```python
from build123d import *

# Parameters (mm, degrees)
FILLET1_R    = 2.1
SCALE1_SCALE = 1.2
SCALE2_SCALE = 0.1


with BuildPart() as part:
    # Sketch1 → Revolve1 (revolve)
    with BuildSketch(Plane.XY):
        with BuildLine():
            Line((-15.5, 65), (15.5, 65))
            Line((15.5, 65), (15.5, 53))
            Line((15.5, 53), (8.94427191, 53))
            ThreePointArc((8.94427191, 53), (0, 57), (-8.94427191, 53))
            Line((-8.94427191, 53), (-15.5, 53))
            Line((-15.5, 53), (-15.5, 65))
        make_face()
    revolve(axis=Axis((-12.809085422, 0, 0), (1, 0, 0)))

    # Fillet1
    fillet1_edges = [part.edges().sort_by_distance(p)[0] for p in [
        (15.5, -65, 0),
        (-15.5, -65, 0),
    ]]
    fillet(fillet1_edges, radius=FILLET1_R)


with BuildPart() as part_1:
    # Scale1: scaled about (0, 0, 0)
    add(part.part.scale(SCALE1_SCALE))


with BuildPart() as part_2:
    # Scale2: scaled about (0, 0, 0)
    add(part_1.part.scale(SCALE2_SCALE))


solid = part_2.part
```
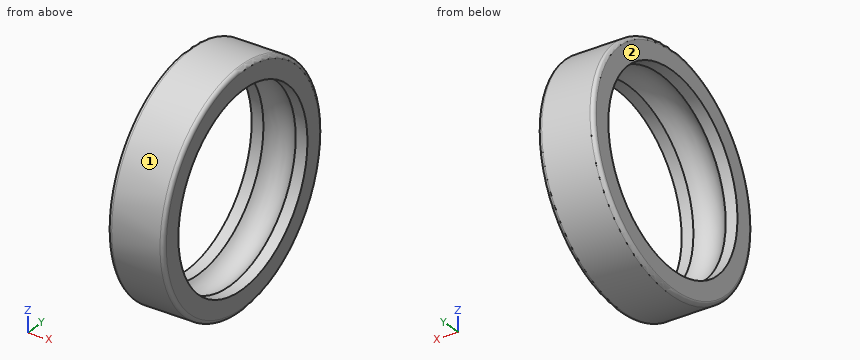
Read the model definition and answer for the solid it produces. Units are mm, in the model's axes. Face numbers are marked on the shaded views. Coordinates: 2 decimals unless noted, no trailing zeros. Write each loop counter-clockwise with the first axis right and the second up, starting at its lowest first coordinate (ties: lowest second). Pieces come first, ordered by that corner, then holes. Notation, with made-up numbers: (11, 35.25) -> (43, 35.25) arc R23 ccw to (43, 59.25) -> close; hole circle Ø11 at (32, -25). An arc over 180 degrees is marked (long way). Return JSON: item names as keys, results as strings.
1. Determine the mould class of the marked faces 1 and 2 for opening direction Z: pulls with the +Z half, pulls with the -Z half, needs draft (parallel to the pull), parting line crosses it, or undercut.
Found:
{"face 1": "parting line crosses it", "face 2": "needs draft"}
2. Find the intervals of material crossed by line 1 along Z through (x, y) = (-1.4, 0); line 2 along Z through (x, y) = (1.6, 1); line 3 along Y through (x, z) = (-0.8, 3), in increasing order. Write a range as from..to.
Found:
{"line 1": "-7.8..-6.36, 6.36..7.8", "line 2": "-7.74..-6.28, 6.28..7.74", "line 3": "-7.2..-5.88, 5.88..7.2"}
3. A cutting plane is placed at A-A (z = 0). Determine the outline of the cut face in (x, y).
Found:
{"outline": "(-1.86, -7.55) arc R0.25 ccw to (-1.61, -7.8) -> (1.61, -7.8) arc R0.25 ccw to (1.86, -7.55) -> (1.86, -6.36) -> (1.07, -6.36) arc R1.44 cw to (-1.07, -6.36) -> (-1.86, -6.36) -> close; (-1.86, 6.36) -> (-1.07, 6.36) arc R1.44 cw to (1.07, 6.36) -> (1.86, 6.36) -> (1.86, 7.55) arc R0.25 ccw to (1.61, 7.8) -> (-1.61, 7.8) arc R0.25 ccw to (-1.86, 7.55) -> close"}
4. A cutting plane is placed at C-C (x = 0). Determine the outline of the cut face in (y, z).
Found:
{"outline": "circle Ø15.6 at (0, 0); hole circle Ø13.68 at (0, 0)"}
5. This flat-tipped pin is pushed along its axis until it touches: P1, Ø1, axis at x = 1, y = 5.5, coming from the +Z side. Where does it stop, or does it pass through?
Found:
{"P1": "z = 5.99"}
